```python
from build123d import *

# Parameters (mm, degrees)
F0_R     = 1.875
F1_DEPTH = 30
F2_DEPTH = 2
F3_START = 28
F3_DEPTH = 2


with BuildPart() as f1:
    # F0 (on Top) → F1 (new body)
    with BuildSketch(Plane.XY):
        Polygon((-10, -17.3205080757), (10, -17.3205080757), (13.25, -11.6913429511), (9.25, -11.6913429511), (14.25, -3.0310889132), (16.25, -6.4951905284), (20, 0), (10, 17.3205080757), (3.5, 17.3205080757), (5.5, 13.8564064606), (-4.5, 13.8564064606), (-2.5, 17.3205080757), (-10, 17.3205080757), (-20, 0), (-16.75, -5.6291651246), (-14.75, -2.1650635095), (-9.75, -10.8253175473), (-13.75, -10.8253175473), align=None)
        Circle(F0_R, mode=Mode.SUBTRACT)
    extrude(amount=F1_DEPTH)

    # F0 (on Top) → F2 (join)
    with BuildSketch(Plane.XY):
        Polygon((-16.75, -5.6291651246), (-13.75, -10.8253175473), (-9.75, -10.8253175473), (-14.75, -2.1650635095), align=None)
        Polygon((9.25, -11.6913429511), (13.25, -11.6913429511), (16.25, -6.4951905284), (14.25, -3.0310889132), align=None)
        Polygon((5.5, 13.8564064606), (3.5, 17.3205080757), (-2.5, 17.3205080757), (-4.5, 13.8564064606), align=None)
    extrude(amount=F2_DEPTH)

    # F0 (on Top) → F3 (join)
    with BuildSketch(Plane.XY.offset(F3_START)):
        Circle(F0_R)
    extrude(amount=F3_DEPTH)


solid = f1.part
```
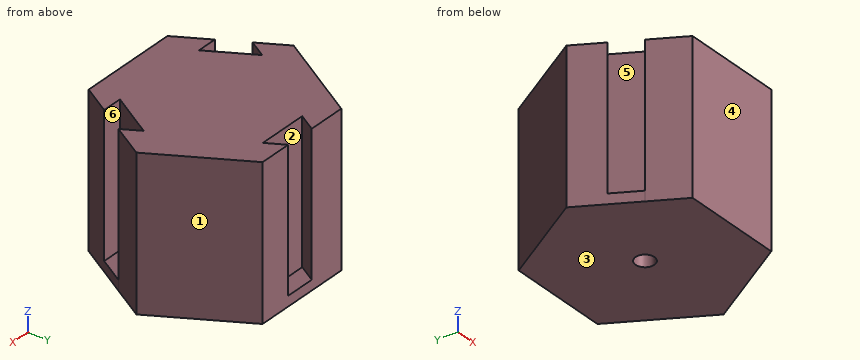
Here's how the part is built. I have some questions about the finished solid (model axes, mm). Face numbers are marked on the shaded views. A direction names the side the tool comes from. Round coordinates to 2 decimals unless told otherwise and drop trailing zeros. Loops run counter-clockwise (first coordinate to the right, second up) from the corner with the lowest first, then second, coordinate; pieces in that order, holes last. Notation, with made-up numbers: (-7, 1) -> (48, 1) arc R9 cw to (48, 11) -> close; hole circle Ø3 at (21, 32.5). An arc over 180 degrees is marked (long way). Answer as CSV lines item,"result".
1. If I drill on L1, parallel to Y at x = 0, z = 18.5 (1 decimal); L2, parallel to Y at x = 12.5, z = 9.75; L3, parallel to X at y = -4.5, z = 18.75, over which ranges is the centre line in solid material (lowest first)?
Final values:
L1,"y = -17.3 to -1.9, 1.9 to 13.9"
L2,"y = -12.99 to -11.69, -6.06 to 12.99"
L3,"x = -17.4 to -16.1, -13.4 to 13.4, 15.1 to 17.4"
2. Thinking about a two-plate mould opening in Y: for the marked faces 1, 2 and 3, which applies, released by +Y, released by -Y, zero draft, split by the parting line, or undercut?
Final values:
face 1,"released by +Y"
face 2,"undercut"
face 3,"zero draft"
3. If we section it at B-B on x = 0: Please give me the cut outline in (y, z) (1 decimal), plus the area to 3 significant figures.
Final values:
outline,"(-17.3, 0) -> (-1.9, 0) -> (-1.9, 28) -> (1.9, 28) -> (1.9, 0) -> (17.3, 0) -> (17.3, 2) -> (13.9, 2) -> (13.9, 30) -> (-17.3, 30) -> close"
area,"837 mm^2"
4. Which directions (+Z, -Z, +X, -X, +Y, -Y) give clear straight access to the entire face, cutting with the end or side of a thin tool? Please do the marked faces 4, 5 and 6.
Final values:
face 4,"+Z, -Z, +X, -X, -Y"
face 5,"+Z"
face 6,"+Z, +X"
5. If we section it at C-C on y = -5: Please give me the cut outline in (x, z), plus the area to 3 significant figures.
Final values:
outline,"(-17.11, 0) -> (17.11, 0) -> (17.11, 30) -> (15.39, 30) -> (15.39, 2) -> (13.11, 2) -> (13.11, 30) -> (-13.11, 30) -> (-13.11, 2) -> (-16.39, 2) -> (-16.39, 30) -> (-17.11, 30) -> close"
area,"871 mm^2"
6. If we section it at D-D on x = 11: Please give me the cut outline in (y, z).
Final values:
outline,"(-15.59, 0) -> (15.59, 0) -> (15.59, 30) -> (-8.66, 30) -> (-8.66, 2) -> (-11.69, 2) -> (-11.69, 30) -> (-15.59, 30) -> close"
7. For pin 1 (4 mm diameter, centred on y = 0.5, z = 15, fed in from -X); pin 2 (3 mm diameter, centred on x = 0, y = 0, fed in from -Z); pin 3 (3 mm diameter, centred on x = -0.5, y = 16.5, fed in from +Z), each with a flat end and sliding along its axis, tell me the tip position at first contact or that it passes through.
Final values:
pin 1,"stops at x = -20"
pin 2,"stops at z = 28"
pin 3,"stops at z = 2"
